Input: part model. Units: mm. Frame: model coordinates. A direction names the side the tool comes from. Coordinates: 2 decimals unless noted, no trailing zeros. Write each loop counter-clockwise with the first axis right and the second up, starting at its lowest first coordinate (ties: lowest second). Pieces come first, ordered by that corner, then holes.
from build123d import *

# Parameters (mm, degrees)
F0_W     = 558.8
F0_H     = 228.6
F1_DEPTH = 19.05
F2_W     = 12.7
F2_H     = 12.7
F3_DEPTH = 558.8
F4_W     = 9.525
F4_H     = 44.45
F4_H_2   = 25.4
F5_DEPTH = 19.05


with BuildPart() as f1:
    # F0 (on Right) → F1 (new body)
    with BuildSketch(Plane.YZ):
        Rectangle(F0_W, F0_H)
    extrude(amount=F1_DEPTH)

    # F2 (on face) → F3 (cut, through all)
    with BuildSketch(Plane.XZ.offset(279.4)):
        with Locations((6.35, 107.95)):
            Rectangle(F2_W, F2_H)
    extrude(amount=-F3_DEPTH, mode=Mode.SUBTRACT)

    # F4 (on face) → F5 (cut, through all)
    with BuildSketch(Plane.YZ.offset(19.05)):
        with Locations((-274.6375, 79.375)):
            Rectangle(F4_W, F4_H)
        with Locations((-274.6375, 31.75)):
            Rectangle(F4_W, F4_H_2)
        with Locations((-274.6375, -6.35)):
            Rectangle(F4_W, F4_H_2)
        with Locations((-274.6375, -44.45)):
            Rectangle(F4_W, F4_H_2)
        with Locations((-274.6375, -92.075)):
            Rectangle(F4_W, F4_H)
        with Locations((274.6375, 79.375)):
            Rectangle(F4_W, F4_H)
        with Locations((274.6375, 31.75)):
            Rectangle(F4_W, F4_H_2)
        with Locations((274.6375, -6.35)):
            Rectangle(F4_W, F4_H_2)
        with Locations((274.6375, -44.45)):
            Rectangle(F4_W, F4_H_2)
        with Locations((274.6375, -92.075)):
            Rectangle(F4_W, F4_H)
    extrude(amount=-F5_DEPTH, mode=Mode.SUBTRACT)


solid = f1.part
Item 1: Section query B-B, the plane z = 65. Return loops of the section in (x, y) (3 decimals).
Item 2: Pin query (flat end, axial travel): pin 1 Ø3 at (x, y) = (6.5, 275) entering from +Z; pin 2 Ø7.5 at (x, y) = (8.5, -274) entering from -Z; pin 3 Ø5 at (x, z) = (14.5, 79.5) entering from +Y (3 decimals). Return the tip coordinate at first contact, or that it passes through.
Item 3: Material intervals for line 1 (Z direction, x = 7.5, y = -160.5); line 2 (Y direction, x = 14, z = -8) (3 decimals), sorted ascending.
Item 4: Section query A-A, the plane y = -108. Return loops of the section in (x, z).
Item 5: Pull-direction query (Z, two-part tool) for faces 5 (the face through (9, 279.4, -64)), 6 (the face through (10, 275, -69.85)), 7 (the face through (10, 269.875, 32)); classes: released by +Z, released by -Z, zero draft, split by the parting line, or undercut.
Item 6: Access query for faces 1 (the face through (10, -269.875, -45)), 2 (the face through (10, -269.875, -92)), 3 (the face through (10, 269.875, 79)), 4 (the face through (10, 269.875, -92)). Directions: +Z, -Z, +X, -X, +Y, -Y. A direction counts if a zero-diameter tool reaches every point of the face in a straight line with its end or side. Return the directions, or none.
The answers:
1. outline: (0, -269.875) - (19.05, -269.875) - (19.05, 269.875) - (0, 269.875) - close
2. pin 1: stops at z = 57.15
2. pin 2: stops at z = -69.85
2. pin 3: stops at y = 269.875
3. line 1: z = -114.3 to 101.6
3. line 2: y = -269.875 to 269.875
4. outline: (0, -114.3) - (19.05, -114.3) - (19.05, 114.3) - (12.7, 114.3) - (12.7, 101.6) - (0, 101.6) - close
5. face 5: zero draft
5. face 6: released by -Z
5. face 7: undercut
6. face 1: +X, -X, -Y
6. face 2: -Z, +X, -X, -Y
6. face 3: +X, -X, +Y
6. face 4: -Z, +X, -X, +Y
